Could you check a few things on this model? Use its own coordinates, in mm. A direction names the side the tool comes from. Give positions to 0.01 mm unless a question says otherwise; leave off trailing zeros. Loops run counter-clockwise (first coordinate to the right, second up) from the corner with the lowest first, then second, coordinate; pieces in that order, holes last. Notation, with made-up numbers: (44.25, 0) - (59.25, 0) arc R33 ccw to (59.25, 34) - close; hole circle Ø5 at (-37.5, 81.5). An arc over 180 degrees is marked (long way). Write each question's results on one line, items separated by ' | '. Start each with the question number.
1) If I drill on probe 1 along Z at (x, y) = (-549, -224); probe 2 along X at (y, z) = (-185, 86); probe 3 along X at (y, z) = (-556.5, 50.5), over which ranges is the centre line in solid material (lowest first)? Write a range as [from, to].
2) I want a section at D-D, the plane z = 108.5. Write out the boundary of the cut face in (x, y).
3) I'm going to push flat-ended pins straight in: pin 1 (22.5 mm diameter, centred on x = 220.29, y = -30.49, fed in from +Z); pin 2 (7.5 mm diameter, centred on x = 218.5, y = -583.5, fed in from -Z); pin 3 (5 mm diameter, centred on y = -187, z = 45, fed in from -X); pin 4 (1.5 mm diameter, centred on x = 170.5, z = 65, fed in from -Y). Where does each tip first touch, or does it pass through?
4) I want a section at B-B, the plane z = 10. Write out the boundary of the cut face in (x, y), and give its area (3 significant figures).
5) I want a section at C-C, the plane x = -455.5. Write out the boundary of the cut face in (y, z), and give its area (3 significant figures).
6) On a 3-axis mill with a long thin cutter (end or side, diameter ignored), from which of +Z, -Z, +X, -X, +Y, -Y can I reach the whole of each face in a straight line? I mean faces 4 (the face through (-516, -319, 153.054)), 5 (the face through (122, -306, -36.946)), 6 (the face through (275, -306, 63.054)). Say none if no direction works.
7) I want a section at A-A, the plane y = -334. Write out the boundary of the cut face in (x, z).
8) If we mould it in two halves opening along Z, with no side actions, what happens to faces 1 (the face through (-507, -306, 163.054)), 2 (the face through (-516, -10, 64)), 3 (the face through (886.031, -306, 12))? For each: +Z half, -Z half, draft (parallel to the pull), parting line (faces both ways), or undercut.
from build123d import *

# Parameters (mm, degrees)
F1_DEPTH = 620
F2_R     = 12.5
F3_DEPTH = 25
F5_DEPTH = 300
F6_W     = 620
F6_H     = 100
F7_DEPTH = 620
F8_R     = 12.5
F9_DEPTH = 25


with BuildPart() as f1:
    # F0 (on Front) → F1 (new body)
    with BuildSketch(Plane.XZ):
        Polygon((266.030722, -36.945744), (266.030722, 63.054256), (-353.969278, 63.054256), (-353.969278, 163.054256), (-663.969278, 163.054256), (-663.969278, -36.945744), (-353.969278, -36.945744), align=None)
    extrude(amount=F1_DEPTH)

    # F2 (on face) → F3 (cut)
    with BuildSketch(Plane(origin=(0, 0, -36.945744), x_dir=(1, 0, 0), z_dir=(0, 0, -1))):
        with Locations((-618.232899, 589.50908)):
            Circle(F2_R)
        with Locations((-618.232899, 30.49092)):
            Circle(F2_R)
        with Locations((220.294342, 589.50908)):
            Circle(F2_R)
        with Locations((220.294342, 30.49092)):
            Circle(F2_R)
    extrude(amount=-F3_DEPTH, mode=Mode.SUBTRACT)

    # F4 (on face) → F5 (cut)
    with BuildSketch(Plane(origin=(-663.969278, 0, 0), x_dir=(0, -1, 0), z_dir=(-1, 0, 0))):
        Polygon((634.776235, 153.054256), (610, 153.054256), (10, 153.054256), (10, -26.945745), (610, -26.945745), (634.776235, -26.945745), align=None)
    extrude(amount=-F5_DEPTH, mode=Mode.SUBTRACT)

    # F6 (on face) → F7 (join, through all)
    with BuildSketch(Plane(origin=(0, 0, 0), x_dir=(-1, 0, 0), z_dir=(0, 1, 0))):
        with Locations((-576.030722, 13.054256)):
            Rectangle(F6_W, F6_H)
    extrude(amount=-F7_DEPTH)

    # F8 (on face) → F9 (cut, through all)
    with BuildSketch(Plane(origin=(0, 0, -36.945744), x_dir=(1, 0, 0), z_dir=(0, 0, -1))):
        with Locations((840.294342, 589.50908)):
            Circle(F8_R)
        with Locations((840.294342, 30.49092)):
            Circle(F8_R)
    extrude(amount=-F9_DEPTH, mode=Mode.SUBTRACT)


solid = f1.part
Answers:
1) probe 1: z = [-36.95, -26.95], [153.05, 163.05] | probe 2: x = [-363.97, -353.97] | probe 3: x = [-363.97, 886.03]
2) outline: (-663.97, -10) - (-363.97, -10) - (-363.97, -620) - (-353.97, -620) - (-353.97, 0) - (-663.97, 0) - close
3) pin 1: stops at z = 63.05 | pin 2: stops at z = -11.95 | pin 3: stops at x = -363.97 | pin 4: passes through
4) outline: (-663.97, -10) - (-363.97, -10) - (-363.97, -620) - (886.03, -620) - (886.03, 0) - (-663.97, 0) - close | area: 778,000 mm2
5) outline: (-620, -36.95) - (0, -36.95) - (0, 163.05) - (-620, 163.05) - (-620, 153.05) - (-10, 153.05) - (-10, -26.95) - (-620, -26.95) - close | area: 14,200 mm2
6) face 4: -X, -Y | face 5: -Z, +X, -X, +Y, -Y | face 6: +Z, +X, +Y, -Y
7) outline: (-663.97, -36.95) - (886.03, -36.95) - (886.03, 63.05) - (-353.97, 63.05) - (-353.97, 163.05) - (-663.97, 163.05) - (-663.97, 153.05) - (-363.97, 153.05) - (-363.97, -26.95) - (-663.97, -26.95) - close
8) face 1: +Z half | face 2: undercut | face 3: draft
